```python
from build123d import *

# Parameters (mm, degrees)
SKETCH_1_R          = 20
SKETCH_1_R_2        = 3
EXTRUDE_1_DEPTH     = 40
SKETCH_2_R          = 3
CUT_EXTRUDE_1_DEPTH = 15


with BuildPart() as part:
    # 草图1 → 凸台-拉伸1 (new body)
    with BuildSketch(Plane(origin=(0, 0, 0), x_dir=(1, 0, 0), z_dir=(0, 1, 0))):
        Polygon((-33, -24), (33, -24), (33, 11), (20, 24), (-20, 24), (-33, 11), align=None)
        with Locations(Location((0, 0, 0), (0, 0, 270))):
            Circle(SKETCH_1_R, mode=Mode.SUBTRACT)
        with Locations(Location((-25.5, 0, 0), (0, 0, 270))):
            Circle(SKETCH_1_R_2, mode=Mode.SUBTRACT)
        with Locations(Location((-18.03122292, 18.03122292, 0), (0, 0, 270))):
            Circle(SKETCH_1_R_2, mode=Mode.SUBTRACT)
        with Locations(Location((-18.03122292, -18.03122292, 0), (0, 0, 270))):
            Circle(SKETCH_1_R_2, mode=Mode.SUBTRACT)
        with Locations(Location((18.03122292, -18.03122292, 0), (0, 0, 90))):
            Circle(SKETCH_1_R_2, mode=Mode.SUBTRACT)
        with Locations(Location((18.03122292, 18.03122292, 0), (0, 0, 90))):
            Circle(SKETCH_1_R_2, mode=Mode.SUBTRACT)
        with Locations(Location((25.5, 0, 0), (0, 0, 90))):
            Circle(SKETCH_1_R_2, mode=Mode.SUBTRACT)
    extrude(amount=EXTRUDE_1_DEPTH)

    # 草图2 → 切除-拉伸1 (cut)
    with BuildSketch(Plane.XY.offset(24)):
        with Locations((-25, 32)):
            Circle(SKETCH_2_R)
        with Locations((-25, 8)):
            Circle(SKETCH_2_R)
        with Locations(Location((25, 8, 0), (0, 0, 180))):
            Circle(SKETCH_2_R)
        with Locations(Location((25, 32, 0), (0, 0, 180))):
            Circle(SKETCH_2_R)
    extrude(amount=-CUT_EXTRUDE_1_DEPTH, mode=Mode.SUBTRACT)


solid = part.part
```
Part model, mm, in its own coordinate system. A direction names the side the tool comes from. Round coordinates to 2 decimals unless told otherwise and drop trailing zeros. Write each loop counter-clockwise with the first axis right and the second up, starting at its lowest first coordinate (ties: lowest second). Pieces come first, ordered by that corner, then holes. Notation, with made-up numbers: M -1,17.5 L 10,17.5 A12 ccw 10,29.5 Z; hole C -8.75,79 d8. An arc over 180 degrees is marked long. One line per question, with ' | ' between items.
(1) Saw through at A-A on x = 0. Write the cut outline in (y, z), then the cut area to 3 significant figures.
Answer key:
outline: M 0,-24 L 40,-24 L 40,-20 L 0,-20 Z; M 0,20 L 40,20 L 40,24 L 0,24 Z | area: 320 mm^2
(2) 3-axis set-ups, long thin cutter, end or side, ignore diameter. For faces 5 (the face through (0, 20, -24)), 6 (the face through (25, 32, 9)): which of +Z, -Z, +X, -X, +Y, -Y reach the whole face in a straight line?
Answer key:
face 5: -Z, +X, -X, +Y, -Y | face 6: +Z
(3) Saw through at B-B on z = 16.5. Write the cut outline in (x, y), then the cut area to 3 significant figures.
Answer key:
outline: M -33,0 L -20.61,0 L -20.61,40 L -33,40 Z; M -15.45,0 L -11.3,0 L -11.3,40 L -15.45,40 Z; M 11.3,0 L 15.45,0 L 15.45,40 L 11.3,40 Z; M 20.61,0 L 33,0 L 33,40 L 20.61,40 Z; hole C -25,8 d6; hole C -25,32 d6; hole C 25,8 d6; hole C 25,32 d6 | area: 1,210 mm^2
(4) Pin check, flat tips, straight feed: pin 1 (6.5 mm diameter, centred on x = -25, y = 7.5, fed in from +Z); pin 2 (5 mm diameter, centred on x = -25, y = 32, fed in from -Z); pin 3 (1.8 mm diameter, centred on x = -26, y = 31, fed in from +Z); pin 4 (9.5 mm diameter, centred on x = -25, y = 8, fed in from -Z). Stop position of each tip, or through.
Answer key:
pin 1: stops at z = 24 | pin 2: stops at z = -21.5 | pin 3: stops at z = 9 | pin 4: stops at z = -23.75
(5) Saw through at D-D on y = 8. Write the cut outline in (x, z).
Answer key:
outline: M -33,-11 L -20,-24 L 20,-24 L 33,-11 L 33,24 L 28,24 L 28,9 L 22,9 L 22,24 L -22,24 L -22,9 L -28,9 L -28,24 L -33,24 Z; hole C -25.5,0 d6; hole C -18.03,-18.03 d6; hole C -18.03,18.03 d6; hole C 0,0 d40; hole C 18.03,-18.03 d6; hole C 18.03,18.03 d6; hole C 25.5,0 d6
(6) Two-plate mould, pull along Y, no slides. Class faces 1 (the face through (0, 0, 21)), 2 (the face through (20.7, 19.7, -19.4)), 3 (the face through (-27.21, 34.03, 16.6)), 4 (the face through (28, 32, 17)): released by +Y, released by -Y, zero draft, split by the parting line, or undercut.
Answer key:
face 1: released by -Y | face 2: zero draft | face 3: undercut | face 4: undercut
(7) Saw through at C-C on z = 0. Write the cut outline in (x, y), then the cut area to 3 significant figures.
Answer key:
outline: M -33,0 L -28.5,0 L -28.5,40 L -33,40 Z; M -22.5,0 L -20,0 L -20,40 L -22.5,40 Z; M 20,0 L 22.5,0 L 22.5,40 L 20,40 Z; M 28.5,0 L 33,0 L 33,40 L 28.5,40 Z | area: 560 mm^2
(8) Probe line 1 along X through (y, z) = (24, 0); line 2 along Y through (x, z) = (-25, 14); line 3 along X through (y, z) = (13, -1.5). List the from-to ranges inside material, lowest first.
Answer key:
line 1: x = -33 to -28.5, -22.5 to -20, 20 to 22.5, 28.5 to 33 | line 2: y = 0 to 5, 11 to 29, 35 to 40 | line 3: x = -33 to -28.1, -22.9 to -19.94, 19.94 to 22.9, 28.1 to 33
